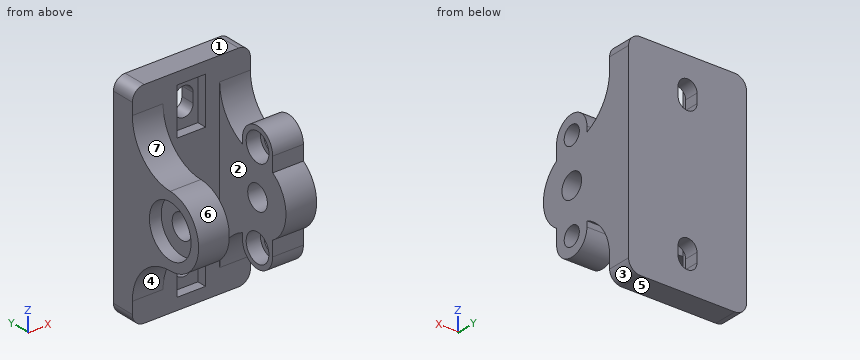
```python
from build123d import *

# Parameters (mm, degrees)
F1_DEPTH  = 5
F2_W      = 6
F2_H      = 10
F3_DEPTH  = 2
F5_START  = 6
F4_R      = 2.6
F5_DEPTH  = 6.5
F6_START  = -6
F6_DEPTH  = 6.5
F7_R      = 5.5
F8_DEPTH  = 2.5
F9_R      = 2
F10_DEPTH = 6.5
F11_R     = 3
F12_DEPTH = 3


with BuildPart() as f1:
    # F0 (on Front) → F1 (new body)
    with BuildSketch(Plane.XZ):
        with BuildLine():
            Line((10, 22.5), (-10, 22.5))
            ThreePointArc((-10, 22.5), (-11.767766953, 21.767766953), (-12.5, 20))
            Line((-12.5, 20), (-12.5, -20))
            ThreePointArc((-12.5, -20), (-11.767766953, -21.767766953), (-10, -22.5))
            Line((-10, -22.5), (10, -22.5))
            ThreePointArc((10, -22.5), (11.767766953, -21.767766953), (12.5, -20))
            Line((12.5, -20), (12.5, 20))
            ThreePointArc((12.5, 20), (11.767766953, 21.767766953), (10, 22.5))
        make_face()
        with BuildLine():
            ThreePointArc((-2, -14), (0, -12), (2, -14))
            Line((2, -14), (2, -16))
            ThreePointArc((2, -16), (0, -18), (-2, -16))
            Line((-2, -16), (-2, -14))
        make_face(mode=Mode.SUBTRACT)
        with BuildLine():
            ThreePointArc((2, 14), (0, 12), (-2, 14))
            Line((-2, 14), (-2, 16))
            ThreePointArc((-2, 16), (0, 18), (2, 16))
            Line((2, 16), (2, 14))
        make_face(mode=Mode.SUBTRACT)
    extrude(amount=F1_DEPTH)

    # F2 (on face) → F3 (cut)
    with BuildSketch(Plane.XZ.offset(5)):
        with Locations((0, 15)):
            Rectangle(F2_W, F2_H)
        with Locations((0, -15)):
            Rectangle(F2_W, F2_H)
    extrude(amount=-F3_DEPTH, mode=Mode.SUBTRACT)

    # F4 (on Right) → F5 (join)
    with BuildSketch(Plane.YZ.offset(F5_START)):
        with BuildLine():
            ThreePointArc((-5, 17.5), (-7.9289321881, 10.4289321881), (-15, 7.5))
            ThreePointArc((-15, 7.5), (-22.5, 0), (-15, -7.5))
            ThreePointArc((-15, -7.5), (-7.9289321881, -10.4289321881), (-5, -17.5))
            Line((-5, -17.5), (-5, 17.5))
        make_face()
        with Locations((-15, 0)):
            Circle(F4_R, mode=Mode.SUBTRACT)
    extrude(amount=F5_DEPTH)

    # F4 (on Right) → F6 (join)
    with BuildSketch(Plane.YZ.offset(F6_START)):
        with BuildLine():
            ThreePointArc((-5, 17.5), (-7.9289321881, 10.4289321881), (-15, 7.5))
            ThreePointArc((-15, 7.5), (-22.5, 0), (-15, -7.5))
            ThreePointArc((-15, -7.5), (-7.9289321881, -10.4289321881), (-5, -17.5))
            Line((-5, -17.5), (-5, 17.5))
        make_face()
        with Locations((-15, 0)):
            Circle(F4_R, mode=Mode.SUBTRACT)
    extrude(amount=-F6_DEPTH)

    # F7 (on face) → F8 (cut)
    with BuildSketch(Plane(origin=(-12.5, 0, 0), x_dir=(0, -1, 0), z_dir=(-1, 0, 0))):
        with Locations((15, 0)):
            Circle(F7_R)
    extrude(amount=-F8_DEPTH, mode=Mode.SUBTRACT)

    # F9 (on face) → F10 (join, through all)
    with BuildSketch(Plane.YZ.offset(12.5)):
        with BuildLine():
            Line((-11, 2.6), (-11, 9.5))
            ThreePointArc((-11, 9.5), (-15, 13.5), (-19, 9.5))
            Line((-19, 9.5), (-19, 2.6))
            Line((-19, 2.6), (-11, 2.6))
        make_face()
        with Locations((-15, 9.5)):
            Circle(F9_R, mode=Mode.SUBTRACT)
        with BuildLine():
            Line((-19, -2.6), (-19, -9.5))
            ThreePointArc((-19, -9.5), (-15, -13.5), (-11, -9.5))
            Line((-11, -9.5), (-11, -2.6))
            Line((-11, -2.6), (-19, -2.6))
        make_face()
        with Locations((-15, -9.5)):
            Circle(F9_R, mode=Mode.SUBTRACT)
    extrude(amount=-F10_DEPTH)

    # F11 (on face) → F12 (cut)
    with BuildSketch(Plane(origin=(6, 0, 0), x_dir=(0, -1, 0), z_dir=(-1, 0, 0))):
        with Locations((15, 9.5)):
            Circle(F11_R)
        with Locations((15, -9.5)):
            Circle(F11_R)
    extrude(amount=-F12_DEPTH, mode=Mode.SUBTRACT)


solid = f1.part
```
For this review, take the finished solid that the model builds, in its own axes (mm). Face numbers are marked on the shaded views. A direction names the side the tool comes from. Coordinates: 2 decimals unless noted, no trailing zeros. Loops run counter-clockwise (first coordinate to the right, second up) from the corner with the lowest first, then second, coordinate; pieces in that order, holes last. Notation, with made-up numbers: (56, -19.5) - (110, -19.5) arc R20 cw to (110, -3.5) - close; hole circle Ø1 at (36, -32). An arc over 180 degrees is marked (long way). Use one line per item in the form item = value. Start each with the question number.
1) Draft analysis for pull direction X (two halves, no side actions). For the marked faces 1, 2 and 3, state which applies: released by +X, released by -X, zero draft, split by the parting line, or undercut.
2) To check wall thickness, follow probe 1 along Z at (x, y) = (6.8, -15); probe 2 along Z at (x, y) = (11.2, -15); probe 3 along X at (y, z) = (-7, -5). State the ranges of each line that lie inside material, in increasing order. Write a range as from..to.
3) Take a section at A-A (y = -7). State the section outline as (x, z) points, plus the area to 3 significant figures.
4) For pin 1 (8 mm diameter, centred on x = 2.5, y = -7, fed in from -Z); pin 2 (1 mm diameter, centred on x = -9, y = -10, fed in from -Z); pin 3 (1.6 mm diameter, centred on x = 8.5, z = 8, fed in from -Y), all flat-tipped, find the tip position at first contact; note any pin that passes through.
5) For the marked faces 4, 5, 6 and 7, list the 3-axis set-ups (+Z, -Z, +X, -X, +Y, -Y) from which the entire face can be reached by the end or side of a thin tool; tool diameter is ignored.
6) Take a section at B-B (x = 0). State the section outline as (y, z) points.
7) Take a section at D-D (x = -9). State the section outline as (y, z) points, plus the area to 3 significant figures.
8) Take a section at C-C (z = 0). State the section outline as (x, y) points, plus the area to 3 significant figures.
From the geometry:
q1.face_1 = zero draft
q1.face_2 = undercut
q1.face_3 = released by +X
q2.probe_1 = -13.5..-12.5, -6.5..-2.6, 2.6..6.5, 12.5..13.5
q2.probe_2 = -13.5..-11.5, -7.5..-2.6, 2.6..7.5, 11.5..13.5
q2.probe_3 = -12.5..-6, 6..12.5
q3.outline = (-12.5, -11.5) - (-6, -11.5) - (-6, 11.5) - (-12.5, 11.5) - close; (6, -11.5) - (12.5, -11.5) - (12.5, 11.5) - (6, 11.5) - close
q3.area = 299 mm2
q4.pin_1 = -22.5
q4.pin_2 = -9.15
q4.pin_3 = -19
q5.face_4 = -Z, -X, -Y
q5.face_5 = -Z, +X, -X, +Y, -Y
q5.face_6 = -X, -Y
q5.face_7 = +Z, -X, -Y
q6.outline = (-5, -22.5) - (0, -22.5) - (0, -18) - (-3, -18) - (-3, -20) - (-5, -20) - close; (-5, -10) - (-3, -10) - (-3, -12) - (0, -12) - (0, 12) - (-3, 12) - (-3, 10) - (-5, 10) - close; (-5, 20) - (-3, 20) - (-3, 18) - (0, 18) - (0, 22.5) - (-5, 22.5) - close
q7.outline = (-15, -7.5) arc R10 cw to (-5, -17.5) - (-5, -22.5) - (0, -22.5) - (0, 22.5) - (-5, 22.5) - (-5, 17.5) arc R10 cw to (-15, 7.5) arc R7.5 ccw to start; hole circle Ø5.2 at (-15, 0)
q7.area = 485 mm2
q8.outline = (-12.5, -22.5) - (-6, -22.5) - (-6, -17.6) - (-10, -17.6) - (-10, -20.5) - (-12.5, -20.5) - close; (-12.5, -9.5) - (-10, -9.5) - (-10, -12.4) - (-6, -12.4) - (-6, -5) - (6, -5) - (6, -12.4) - (12.5, -12.4) - (12.5, 0) - (-12.5, 0) - close; (6, -22.5) - (12.5, -22.5) - (12.5, -17.6) - (6, -17.6) - close
q8.area = 270 mm2
